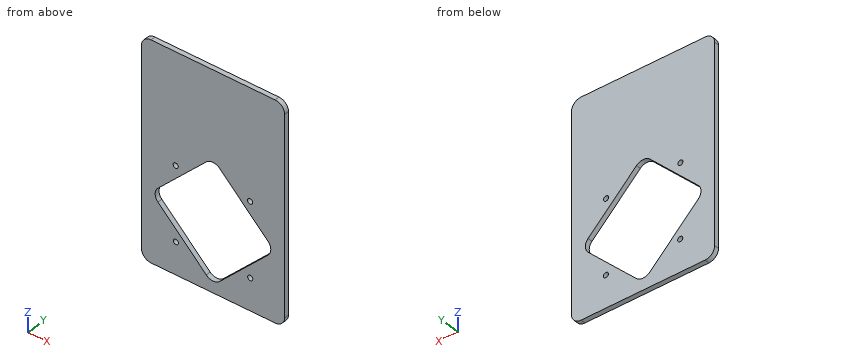
```python
from build123d import *

# Parameters (mm, degrees)
SKETCH1_W           = 94.832
SKETCH1_H           = 144.105
SKETCH1_R           = 1.7
BOSS_EXTRUDE2_DEPTH = 3.175
FILLET1_R           = 6.35
FILLET2_R           = 6.35


with BuildPart() as part:
    # Sketch1 → Boss-Extrude2 (new body)
    with BuildSketch(Plane(origin=(0, 0, 0), x_dir=(1, 0, 0), z_dir=(0, 1, 0))):
        with Locations((47.416, 66.438639868)):
            Rectangle(SKETCH1_W, SKETCH1_H)
        with Locations(Location((22.7875, 117.150797893, 0), (0, 0, 270))):
            Circle(SKETCH1_R, mode=Mode.SUBTRACT)
        with Locations(Location((72.0445, 117.150797893, 0), (0, 0, 270))):
            Circle(SKETCH1_R, mode=Mode.SUBTRACT)
        with Locations(Location((71.919698828, 67.768996721, 0), (0, 0, 270))):
            Circle(SKETCH1_R, mode=Mode.SUBTRACT)
        with Locations(Location((22.662698828, 67.893797893, 0), (0, 0, 270))):
            Circle(SKETCH1_R, mode=Mode.SUBTRACT)
        Polygon((6.429841975, 92.522297893), (47.416, 133.383654746), (88.277356853, 92.397496721), (47.291198828, 51.536139868), align=None, mode=Mode.SUBTRACT)
    extrude(amount=BOSS_EXTRUDE2_DEPTH)

    # Fillet1
    fillet1_edges = [part.edges().sort_by_distance(p)[0] for p in [
        (47.416, 1.5875, -133.383654746),
        (6.429841975, 1.5875, -92.522297893),
        (47.291198828, 1.5875, -51.536139868),
        (88.277356853, 1.5875, -92.397496721),
    ]]
    fillet(fillet1_edges, radius=FILLET1_R)

    # Fillet2
    fillet2_edges = [part.edges().sort_by_distance(p)[0] for p in [
        (94.832, 1.5875, 5.613860132),
        (0, 1.5875, 5.613860132),
        (0, 1.5875, -138.491139868),
        (94.832, 1.5875, -138.491139868),
    ]]
    fillet(fillet2_edges, radius=FILLET2_R)


solid = part.part
```
Verification items for the finished model (mm, model axes). Give positions to 0.01 mm unless a question says otherwise; leave off trailing zeros. Order: outer loops, then holes, each group sorted by start corner. A loop starts at its lowest first (then second) coordinate and runs counter-clockwise, first axis right, second up. Notation, with made-up numbers: (84, -29) -> (120, -29) arc R13 cw to (120, -17) -> close; hole circle Ø3 at (57.25, 7). An arc over 180 degrees is marked (long way). Use a Markdown table: item, result.
1) Depth check by flat-ended pin: pin 1 Ø4.5 at (x, z) = (72.04, -117.15) entering from +Y (3 decimals). Enter the tip coordinate at first touch or a pass-through.
Results:
| item | result |
|---|---|
| pin 1 | y = 3.175 |
2) Material ranges on probe 1 along X at (y, z) = (2.05, -74.5); probe 2 along X at (y, z) = (0.6, -68.5); probe 3 along Z at (x, y) = (66, 0.5), recorded low to high.
Results:
| item | result |
|---|---|
| probe 1 | 0 to 24.4, 70.33 to 94.83 |
| probe 2 | 0 to 21.07, 24.25 to 30.38, 64.31 to 70.38, 73.45 to 94.83 |
| probe 3 | -138.49 to -114.74, -70.19 to 5.61 |
3) Section check A-A, the plane x = 58. Record the boundary of the cut face in (y, z) (3 decimals).
Results:
| item | result |
|---|---|
| outline | (0, -138.491) -> (3.175, -138.491) -> (3.175, -122.767) -> (0, -122.767) -> close; (0, -62.212) -> (3.175, -62.212) -> (3.175, 5.614) -> (0, 5.614) -> close |
4) Section check B-B, the plane z = -92. Record the boundary of the cut face in (x, y) (3 decimals).
Results:
| item | result |
|---|---|
| outline | (0, 0) -> (9.08, 0) -> (9.08, 3.175) -> (0, 3.175) -> close; (85.634, 0) -> (94.832, 0) -> (94.832, 3.175) -> (85.634, 3.175) -> close |
5) Section check C-C, the plane y = 1.45. Record the boundary of the cut face in (x, z).
Results:
| item | result |
|---|---|
| outline | (0, -132.14) arc R6.35 ccw to (6.35, -138.49) -> (88.48, -138.49) arc R6.35 ccw to (94.83, -132.14) -> (94.83, -0.74) arc R6.35 ccw to (88.48, 5.61) -> (6.35, 5.61) arc R6.35 ccw to (0, -0.74) -> close; hole (10.91, -88.03) arc R6.35 ccw to (10.93, -97.01) -> (42.92, -128.9) arc R6.35 ccw to (51.9, -128.89) -> (83.79, -96.89) arc R6.35 ccw to (83.78, -87.91) -> (51.79, -56.02) arc R6.35 ccw to (42.81, -56.03) -> close; hole circle Ø3.4 at (22.66, -67.89); hole circle Ø3.4 at (22.79, -117.15); hole circle Ø3.4 at (71.92, -67.77); hole circle Ø3.4 at (72.04, -117.15) |
